Can you work these out from the model? Positions are in its coordinate system, mm. Coordinates: 2 decimals unless noted, no trailing zeros. Order: outer loops, then holes, each group sorted by start corner. A loop starts at its lowest first (then second) coordinate and runs counter-clockwise, first axis right, second up. Notation, with made-up numbers: (76.5, 67.25) -> (101.5, 67.25) arc R14 cw to (101.5, 82.25) -> close; hole circle Ø11 at (62.5, 76). An arc over 180 degrees is marked (long way). Use a Markdown table: item, result. Add a question column.
1. Suppose I cut it at A-A, the plane x = 0. List the corners of the cut face in (y, z) for me.
2. Suppose I cut it at B-B, the plane z = 1.85. List the corners of the cut face in (x, y) for me.
3. If I drill on line 1 along Y through (x, z) = (0, 3.25); line 2 along Y through (x, z) = (1.25, 0.2); line 3 along X through (y, z) = (1.5, 1), over which ranges is the centre line in solid material (lowest first)? Write a range as from..to.
4. We'd pull the mould along Y, two halves only. Please class faces 1 (the cylindrical face through (-0.456, 1.485, 3.09)), 2 (the cylindrical face through (-4.054, 1.238, 3.11)), 3 (the flat face through (-2, 2, -0.025)): pulls with the +Y half, pulls with the -Y half, needs draft (parallel to the pull), parting line crosses it, or undercut.
5. Suppose I cut it at C-C, the plane z = 3.5. List the corners of the cut face in (x, y) for me.
6. For pin 1 Ø1 at (y, z) = (6.5, 2) entering from +X; pin 2 Ø2 at (y, z) = (7, 2) entering from -X; pin 3 Ø6 at (x, y) = (1.5, 9) entering from -Z; pin 4 Ø1.5 at (x, z) = (-3, 1.5) entering from +Y, each with a flat end and sliding along its axis, tell me the tip position at first contact or that it passes through.
```python
from build123d import *


with BuildPart() as part:
    # Sketch2 → Revolve1 (revolve)
    with BuildSketch(Plane(origin=(0, 0, 0), x_dir=(0, 0, -1), z_dir=(1, 0, 0)), mode=Mode.PRIVATE) as revolve1_sk:
        with BuildLine():
            Line((0.024688303, 1.555426785), (0.024688303, 1.055426785))
            Line((0.024688303, 1.055426785), (-1.341325441, 0.598364979))
            ThreePointArc((-1.341325441, 0.598364979), (-1.436030164, 0.45504575), (-1.341325441, 0.31172652))
            Line((-1.341325441, 0.31172652), (0.024688303, -0.145335285))
            Line((0.024688303, -0.145335285), (0.024688303, -0.644573215))
            Line((0.024688303, -0.644573215), (-0.775311697, -1.044573215))
            Line((-0.775311697, -1.044573215), (-2.375311697, -0.54495425))
            Line((-2.375311697, -0.54495425), (-3.825311697, -0.54495425))
            Line((-3.825311697, -0.54495425), (-3.975311697, -0.34495425))
            Line((-3.975311697, -0.34495425), (-3.975311697, 1.25504575))
            Line((-3.975311697, 1.25504575), (-3.825311697, 1.45504575))
            Line((-3.825311697, 1.45504575), (-2.375311697, 1.45504575))
            Line((-2.375311697, 1.45504575), (-0.7754582, 1.955133643))
            Line((-0.7754582, 1.955133643), (0.024688303, 1.555426785))
        make_face()
    revolve(revolve1_sk.sketch.rotate(Axis((0, 4.955426785, 17.313384256), (0, 0, -1)), 270), axis=Axis((0, 4.955426785, 17.313384256), (0, 0, -1)))


solid = part.part
```
Worked out:
| question | item | result |
|---|---|---|
| 1 | outline | (-1.04, 0.78) -> (-0.64, -0.02) -> (-0.15, -0.02) -> (0.31, 1.34) arc R0.16 cw to (0.6, 1.34) -> (1.06, -0.02) -> (1.56, -0.02) -> (1.96, 0.78) -> (1.46, 2.38) -> (1.46, 3.83) -> (1.26, 3.98) -> (-0.34, 3.98) -> (-0.54, 3.83) -> (-0.54, 2.38) -> close; (7.96, 0.78) -> (8.36, -0.02) -> (8.86, -0.02) -> (9.31, 1.34) arc R0.16 cw to (9.6, 1.34) -> (10.06, -0.02) -> (10.56, -0.02) -> (10.96, 0.78) -> (10.46, 2.38) -> (10.46, 3.83) -> (10.26, 3.98) -> (8.66, 3.98) -> (8.46, 3.83) -> (8.46, 2.38) -> close |
| 2 | outline | circle Ø11.33 at (0, 4.96); hole circle Ø6.67 at (0, 4.96) |
| 3 | line 1 | y = -0.54..1.46, 8.46..10.46 |
| 3 | line 2 | y = -0.62..0.09, 1.18..1.91, 8..8.73, 9.82..10.53 |
| 3 | line 3 | x = -4.82..-3.27, -2.46..2.46, 3.27..4.82 |
| 4 | face 1 | undercut |
| 4 | face 2 | parting line crosses it |
| 4 | face 3 | needs draft |
| 5 | outline | circle Ø11 at (0, 4.96); hole circle Ø7 at (0, 4.96) |
| 6 | pin 1 | stops at x = 5.61 |
| 6 | pin 2 | stops at x = -5.69 |
| 6 | pin 3 | stops at z = -0.02 |
| 6 | pin 4 | stops at y = 10.36 |
